Read the model definition and answer for the solid it produces. Units are mm, in the model's axes. A direction names the side the tool comes from. Coordinates: 2 decimals unless noted, no trailing zeros. Order: outer loops, then holes, each group sorted by start corner. A loop starts at its lowest first (then second) coordinate and runs counter-clockwise, first axis right, second up. Notation, with made-up numbers: M 33,55.25 L 46,55.25 A33 ccw 46,88.25 Z; hole C 50.5,10 d9. An arc over 180 degrees is marked long. Put each result on its own line as item: value.
from build123d import *

# Parameters (mm, degrees)
SKETCH006_W     = 162
SKETCH006_H     = 48
PAD005_DEPTH    = 0.8
PAD006_DEPTH    = 157
POCKET001_DEPTH = 41.5


with BuildPart() as part:
    # Sketch006 → Pad005 (new body)
    with BuildSketch(Plane.YZ):
        with Locations((-78, 19)):
            Rectangle(SKETCH006_W, SKETCH006_H)
    extrude(amount=-PAD005_DEPTH)

    # Sketch007 (on DatumPlane) → Pad006 (join)
    with BuildSketch(Plane.ZX):
        Polygon((1.5, 0), (43, 0), (43, 41.25), (40.5, 41.25), (37.502441, 58.25), (23, 58.25), (20.707749, 71.25), (1.5, 71.25), align=None)
    extrude(amount=-PAD006_DEPTH)

    # Sketch008 (on Face5 of Pad006) → Pocket001 (cut)
    with BuildSketch(Plane(origin=(0, 0, 43), x_dir=(0, -1, 0), z_dir=(0, 0, 1))):
        Polygon((0, 25), (12, 25), (12, 27.5), (31.5, 71.75), (0, 71.75), align=None)
        Polygon((157, 22.75), (157, 71.25), (120, 71.25), (130, 61.25), (130, 41.25), (153.5, 41.25), (153.5, 26.25), align=None)
    extrude(amount=-POCKET001_DEPTH, mode=Mode.SUBTRACT)


solid = part.part
Q1. Find section B-B on y = -75. Write down the section's boundary in (x, z), plus the area to 3 significant figures.
Answers below:
outline: M -0.8,-5 L 0,-5 L 0,1.5 L 71.25,1.5 L 71.25,20.71 L 58.25,23 L 58.25,37.5 L 41.25,40.5 L 41.25,43 L -0.8,43 Z
area: 2,650 mm^2
Q2. Find section A-A on z = 6. Write down the section's boundary in (x, y).
Answers below:
outline: M -0.8,-159 L 0,-159 L 0,-157 L 22.75,-157 L 26.25,-153.5 L 41.25,-153.5 L 41.25,-130 L 61.25,-130 L 71.25,-120 L 71.25,-31.28 L 27.5,-12 L 25,-12 L 25,0 L 0,0 L 0,3 L -0.8,3 Z
Q3. Given pin 1 (4 mm diameter, centred on x = 28.5, y = -126.5, fed in from -Z); pin 2 (12 mm diameter, centred on x = 33, z = 31, fed in from -Y); pin 3 (12 mm diameter, centred on x = 59, y = -98, fed in from +Z), each flat-ended and moving along its own axis, determine where each tip first touches the part or whether it passes through.
Answers below:
pin 1: stops at z = 1.5
pin 2: stops at y = -153.5
pin 3: stops at z = 38.43
Q4. Find section C-C on x = 11.5. Write down the section's boundary in (y, z).
Answers below:
outline: M -157,1.5 L 0,1.5 L 0,43 L -157,43 Z
Q5. A tool of negligible diameter and unlimited length cuts with its end or side. For faces 1 (the face through (34, -153.5, 23)), 2 (the face through (41.25, -131, 27)), 3 (the face through (58.25, -77, 30)), 4 (the face through (36, -77, 1.5)), 5 (the face through (25, -6, 23)), from which of +Z, -Z, +X, -X, +Y, -Y can it reach the whole face along a straight path? Write none if from no direction.
Answers below:
face 1: +Z, -Z, +X, -Y
face 2: +Z, +X, -Y
face 3: +Z, +X, +Y, -Y
face 4: -Z, +X, +Y, -Y
face 5: +Z, -Z, +X, +Y
Q6. Consider line 1 along X through (y, z) = (-104, -1); line 2 along Z through (x, y) = (5.5, -40); line 3 along Y through (x, z) = (4, 9.5). Determine where each line is inside the solid, lowest interval first.
Answers below:
line 1: x = -0.8 to 0
line 2: z = 1.5 to 43
line 3: y = -157 to 0
Q7. For a pull along X with two mould halves and no side action, classify faces 6 (the face through (49.631, -73.246, 39.022)), 7 (the face through (-0.8, -79, 19)), 8 (the face through (12, -157, 22)) as +X half, -X half, draft (parallel to the pull), parting line (faces both ways), or undercut.
Answers below:
face 6: +X half
face 7: -X half
face 8: draft
Q8. Find section D-D on y = -22. Write down the section's boundary in (x, z).
Answers below:
outline: M -0.8,-5 L 0,-5 L 0,1.5 L 50.19,1.5 L 50.19,38.92 L 41.25,40.5 L 41.25,43 L -0.8,43 Z
